from build123d import *

# Parameters (mm, degrees)
F0_R     = 2
F1_DEPTH = 20
F2_R     = 15
F3_DEPTH = 3


with BuildPart() as f1:
    # F0 (on Front) → F1 (new body)
    with BuildSketch(Plane.XZ):
        with BuildLine():
            ThreePointArc((10.134032, -2.650853), (10.389408, -1.336346), (10.475, 0))
            ThreePointArc((10.475, 0), (10.47218, 0.243036), (10.463722, 0.485942))
            ThreePointArc((10.463722, 0.485942), (10.417617, 1.094936), (10.336098, 1.700207))
            ThreePointArc((10.336098, 1.700207), (9.962317, 3.236953), (9.361436, 4.699909))
            ThreePointArc((9.361436, 4.699909), (9.071616, 5.2375), (8.750959, 5.757286))
            ThreePointArc((8.750959, 5.757286), (7.784442, 7.009143), (6.640472, 8.10122))
            ThreePointArc((6.640472, 8.10122), (6.157051, 8.474453), (5.652699, 8.818878))
            ThreePointArc((5.652699, 8.818878), (4.260566, 9.569389), (2.77131, 10.101756))
            ThreePointArc((2.77131, 10.101756), (2.177875, 10.246096), (1.577037, 10.355606))
            ThreePointArc((1.577037, 10.355606), (0, 10.475), (-1.577037, 10.355606))
            ThreePointArc((-1.577037, 10.355606), (-2.177875, 10.246096), (-2.77131, 10.101756))
            ThreePointArc((-2.77131, 10.101756), (-4.260566, 9.569389), (-5.652699, 8.818878))
            ThreePointArc((-5.652699, 8.818878), (-6.157051, 8.474453), (-6.640472, 8.10122))
            ThreePointArc((-6.640472, 8.10122), (-7.784442, 7.009143), (-8.750959, 5.757286))
            ThreePointArc((-8.750959, 5.757286), (-9.071616, 5.2375), (-9.361436, 4.699909))
            ThreePointArc((-9.361436, 4.699909), (-9.962317, 3.236953), (-10.336098, 1.700207))
            ThreePointArc((-10.336098, 1.700207), (-10.417617, 1.094936), (-10.463722, 0.485942))
            ThreePointArc((-10.463722, 0.485942), (-10.417617, -1.094936), (-10.134032, -2.650853))
            ThreePointArc((-10.134032, -2.650853), (-9.962317, -3.236953), (-9.756736, -3.812049))
            ThreePointArc((-9.756736, -3.812049), (-9.071616, -5.2375), (-8.1797, -6.543557))
            ThreePointArc((-8.1797, -6.543557), (-7.784442, -7.009143), (-7.362722, -7.450903))
            ThreePointArc((-7.362722, -7.450903), (-6.157051, -8.474453), (-4.811023, -9.30482))
            ThreePointArc((-4.811023, -9.30482), (-4.260566, -9.569389), (-3.695626, -9.801427))
            ThreePointArc((-3.695626, -9.801427), (-2.177875, -10.246096), (-0.610477, -10.457196))
            ThreePointArc((-0.610477, -10.457196), (0, -10.475), (0.610477, -10.457196))
            ThreePointArc((0.610477, -10.457196), (2.177875, -10.246096), (3.695626, -9.801427))
            ThreePointArc((3.695626, -9.801427), (4.260566, -9.569389), (4.811023, -9.30482))
            ThreePointArc((4.811023, -9.30482), (6.157051, -8.474453), (7.362722, -7.450903))
            ThreePointArc((7.362722, -7.450903), (7.784442, -7.009143), (8.1797, -6.543557))
            ThreePointArc((8.1797, -6.543557), (9.071616, -5.2375), (9.756736, -3.812049))
            ThreePointArc((9.756736, -3.812049), (9.962317, -3.236953), (10.134032, -2.650853))
        make_face()
        Circle(F0_R, mode=Mode.SUBTRACT)
        with BuildLine():
            ThreePointArc((10.463722, 0.485942), (10.47218, 0.243036), (10.475, 0))
            ThreePointArc((10.475, 0), (10.389408, -1.336346), (10.134032, -2.650853))
            Line((10.134032, -2.650853), (11.615503, -2.468951))
            Line((11.615503, -2.468951), (11.875, 0))
            Line((11.875, 0), (10.463722, 0.485942))
        make_face()
        with BuildLine():
            ThreePointArc((9.361436, 4.699909), (9.962317, 3.236953), (10.336098, 1.700207))
            Line((10.336098, 1.700207), (11.615503, 2.468951))
            Line((11.615503, 2.468951), (10.848352, 4.829998))
            Line((10.848352, 4.829998), (9.361436, 4.699909))
        make_face()
        with BuildLine():
            Line((10.848352, -4.829998), (9.756736, -3.812049))
            ThreePointArc((9.756736, -3.812049), (9.071616, -5.2375), (8.1797, -6.543557))
            Line((8.1797, -6.543557), (9.607077, -6.97995))
            Line((9.607077, -6.97995), (10.848352, -4.829998))
        make_face()
        with BuildLine():
            ThreePointArc((6.640472, 8.10122), (7.784442, 7.009143), (8.750959, 5.757286))
            Line((8.750959, 5.757286), (9.607077, 6.97995))
            Line((9.607077, 6.97995), (7.945926, 8.824845))
            Line((7.945926, 8.824845), (6.640472, 8.10122))
        make_face()
        with BuildLine():
            Line((7.945926, -8.824845), (7.362722, -7.450903))
            ThreePointArc((7.362722, -7.450903), (6.157051, -8.474453), (4.811023, -9.30482))
            Line((4.811023, -9.30482), (5.9375, -10.284052))
            Line((5.9375, -10.284052), (7.945926, -8.824845))
        make_face()
        with BuildLine():
            ThreePointArc((2.77131, 10.101756), (4.260566, 9.569389), (5.652699, 8.818878))
            Line((5.652699, 8.818878), (5.9375, 10.284052))
            Line((5.9375, 10.284052), (3.669577, 11.293796))
            Line((3.669577, 11.293796), (2.77131, 10.101756))
        make_face()
        with BuildLine():
            Line((3.669577, -11.293796), (3.695626, -9.801427))
            ThreePointArc((3.695626, -9.801427), (2.177875, -10.246096), (0.610477, -10.457196))
            Line((0.610477, -10.457196), (1.241276, -11.809948))
            Line((1.241276, -11.809948), (3.669577, -11.293796))
        make_face()
        with BuildLine():
            ThreePointArc((-1.577037, 10.355606), (0, 10.475), (1.577037, 10.355606))
            Line((1.577037, 10.355606), (1.241276, 11.809948))
            Line((1.241276, 11.809948), (-1.241276, 11.809948))
            Line((-1.241276, 11.809948), (-1.577037, 10.355606))
        make_face()
        with BuildLine():
            Line((-1.241276, -11.809948), (-0.610477, -10.457196))
            ThreePointArc((-0.610477, -10.457196), (-2.177875, -10.246096), (-3.695626, -9.801427))
            Line((-3.695626, -9.801427), (-3.669577, -11.293796))
            Line((-3.669577, -11.293796), (-1.241276, -11.809948))
        make_face()
        with BuildLine():
            ThreePointArc((-5.652699, 8.818878), (-4.260566, 9.569389), (-2.77131, 10.101756))
            Line((-2.77131, 10.101756), (-3.669577, 11.293796))
            Line((-3.669577, 11.293796), (-5.9375, 10.284052))
            Line((-5.9375, 10.284052), (-5.652699, 8.818878))
        make_face()
        with BuildLine():
            Line((-5.9375, -10.284052), (-4.811023, -9.30482))
            ThreePointArc((-4.811023, -9.30482), (-6.157051, -8.474453), (-7.362722, -7.450903))
            Line((-7.362722, -7.450903), (-7.945926, -8.824845))
            Line((-7.945926, -8.824845), (-5.9375, -10.284052))
        make_face()
        with BuildLine():
            ThreePointArc((-8.750959, 5.757286), (-7.784442, 7.009143), (-6.640472, 8.10122))
            Line((-6.640472, 8.10122), (-7.945926, 8.824845))
            Line((-7.945926, 8.824845), (-9.607077, 6.97995))
            Line((-9.607077, 6.97995), (-8.750959, 5.757286))
        make_face()
        with BuildLine():
            Line((-9.607077, -6.97995), (-8.1797, -6.543557))
            ThreePointArc((-8.1797, -6.543557), (-9.071616, -5.2375), (-9.756736, -3.812049))
            Line((-9.756736, -3.812049), (-10.848352, -4.829998))
            Line((-10.848352, -4.829998), (-9.607077, -6.97995))
        make_face()
        with BuildLine():
            ThreePointArc((-10.336098, 1.700207), (-9.962317, 3.236953), (-9.361436, 4.699909))
            Line((-9.361436, 4.699909), (-10.848352, 4.829998))
            Line((-10.848352, 4.829998), (-11.615503, 2.468951))
            Line((-11.615503, 2.468951), (-10.336098, 1.700207))
        make_face()
        with BuildLine():
            Line((-11.615503, -2.468951), (-10.134032, -2.650853))
            ThreePointArc((-10.134032, -2.650853), (-10.417617, -1.094936), (-10.463722, 0.485942))
            Line((-10.463722, 0.485942), (-11.875, 0))
            Line((-11.875, 0), (-11.615503, -2.468951))
        make_face()
    extrude(amount=F1_DEPTH)

    # F2 (on Front) → F3 (join)
    with BuildSketch(Plane.XZ):
        Circle(F2_R)
    extrude(amount=-F3_DEPTH)


solid = f1.part
For this review, take the finished solid that the model builds, in its own axes (mm). A direction names the side the tool comes from. Give positions to 0.01 mm unless a question says otherwise; leave off trailing zeros. Loops run counter-clockwise (first coordinate to the right, second up) from the corner with the lowest first, then second, coordinate; pieces in that order, holes last. Notation, with made-up numbers: M 82.25,50.5 L 115.25,50.5 A12 ccw 115.25,60.5 Z; hole C -31.5,51 d9. An arc over 180 degrees is marked long. Answer as a JSON object with one key per item and string values. Group by question number.
Q1. Add section A-A on x = 0. Give the boundary of the cut face in (y, z) (3 decimals).
Q2. Mouldability with a two-part tool opening along X and no side actions: class faces 4 (the flat face through (-5.797, -9.86, 9.562)), 5 (the cylindrical face through (10.42, -9.86, 1.09)), 6 (the flat face through (-10.094, -9.86, 4.764)) as +X half, -X half, draft (parallel to the pull), parting line (faces both ways), or undercut.
Q3. Add section B-B on z = -1.5. Give the boundary of the cut face in (x, y).
Q4. Add section C-C on y = 0.5. Give the boundary of the cut face in (x, z), and give its area (3 significant figures).
Q5. Tool access review of faces 1 (the flat face through (-8.903, -9.86, -6.765)), 2 (the flat face through (-6.96, -9.86, -9.54)), 3 (the flat face through (9.2, -9.9, 6.4)): name each direction out of +Z, -Z, +X, -X, +Y, -Y from which nothing blocks a thin tool from reaching the whole face with its end or side.
Q6. For probe 1 along Y at (x, z) = (-4, 13); probe 2 along X at (y, z) = (-2.75, 5.75); probe 3 along Z at (x, y) = (-4.5, -3.25), list the stretches that pass through material, from the lowest coordinate up. Write a range as [from, to].
Q7. Insertion check: P1, Ø8, axis at y = -8.5, z = -9, coming from the -X side; P2, Ø5, axis at y = -8.5, z = 8.5, coming from the -X side; P3, Ø3, axis at x = 4, y = -17.5, coming from the +Z side. Each pin has a flat end and moves straight along its axis. Give the tip position at first contact, or say it passes through.
Checked values:
{
 "1": {"outline": "M -20,-10.475 L 0,-10.475 L 0,-15 L 3,-15 L 3,15 L 0,15 L 0,11.81 L -20,11.81 L -20,2 L 0,2 L 0,-2 L -20,-2 Z"},
 "2": {"face 4": "-X half", "face 5": "+X half", "face 6": "undercut"},
 "3": {"outline": "M -14.92,0 L -11.72,0 L -11.72,-20 L -1.32,-20 L -1.32,0 L 1.32,0 L 1.32,-20 L 11.72,-20 L 11.72,0 L 14.92,0 L 14.92,3 L -14.92,3 Z"},
 "4": {"outline": "C 0,0 d30", "area": "707 mm²"},
 "5": {"face 1": "-Z, -Y", "face 2": "-Z, -X, -Y", "face 3": "+X, -Y"},
 "6": {"probe 1": "[0, 3]", "probe 2": "[-8.76, 8.76]", "probe 3": "[-9.46, 10.92]"},
 "7": {"P1": "x = -10.75", "P2": "x = -9.61", "P3": "z = 11.29"}
}
